from build123d import *

# Parameters (mm, degrees)
SKETCH1_W               = 44.45
SKETCH1_H               = 63.5
BOSS_EXTRUDE1_DEPTH     = 6.35
F_1_4_CLEARANCE_HOLE1_D = 6.7564
F_1_4_CLEARANCE_HOLE3_D = 6.5278


with BuildPart() as part:
    # Sketch1 → Boss-Extrude1 (new body)
    with BuildSketch(Plane(origin=(0, 0, 0), x_dir=(1, 0, 0), z_dir=(0, 1, 0))):
        Rectangle(SKETCH1_W, SKETCH1_H)
    extrude(amount=BOSS_EXTRUDE1_DEPTH)

    # 1/4 Clearance Hole1 (through all)
    with Locations(Plane(origin=(0, 6.35, 0), x_dir=(1, 0, 0), z_dir=(0, 1, 0))):
        with Locations((0, 25.4), (0, 0)):
            Hole(F_1_4_CLEARANCE_HOLE1_D / 2)

    # 1/4 Clearance Hole3 (through all)
    with Locations(Plane(origin=(0, 6.35, 0), x_dir=(1, 0, 0), z_dir=(0, 1, 0))):
        with Locations((-12.7, -22.86), (12.7, -22.86)):
            Hole(F_1_4_CLEARANCE_HOLE3_D / 2)


solid = part.part
Model file for the job. Use its own axes, mm. Give positions to 0.01 mm unless a question says otherwise; leave off trailing zeros. Write each loop counter-clockwise with the first axis right and the second up, starting at its lowest first coordinate (ties: lowest second). Pieces come first, ordered by that corner, then holes. Notation, with made-up numbers: M -11.5,70.25 L 23.5,70.25 A23 ccw 23.5,86.25 Z; hole C 53.25,4.5 d1. An arc over 180 degrees is marked long. One line per item, written item: value. Start each with the question number.
Q1. Saw through at D-D, the plane x = 0. Write the cut outline in (y, z).
Q2. Saw through at C-C, the plane y = 1.25. Write the cut outline in (x, z) (3 decimals), plus the area to 3 significant figures.
Q3. Drop a flat-ended pin along its axis: pin 1 Ø7.5 at (x, z) = (12.7, 22.86) entering from -Y. Give the stop position or say it passes through.
Q4. Two-plate mould, pull along Z, no slides. Class faces 1 (the cylindrical face through (2.681, 3.131, 2.056)), 2 (the flat face through (-5, 6.35, 0)), 3 (the flat face through (0, 3, -31.75)): +Z half, -Z half, draft (parallel to the pull), parting line (faces both ways), or undercut.
Q5. Saw through at B-B, the plane x = -12.7. Write the cut outline in (y, z).
Q6. Saw through at A-A, the plane z = -25.4. Write the cut outline in (x, y) (3 decimals), plus the area to 3 significant figures.
Q7. Probe probe 1 along X at (y, z) = (1.75, 22.86) (3 decimals); probe 2 along Z at (x, y) = (0, 3.5); probe 3 along X at (y, z) = (3, -25.4) (3 decimals). List the from-to ranges inside material, lowest first. Write a range as [from, to].
Output values:
1. outline: M 0,-31.75 L 6.35,-31.75 L 6.35,-28.78 L 0,-28.78 Z; M 0,-22.02 L 6.35,-22.02 L 6.35,-3.38 L 0,-3.38 Z; M 0,3.38 L 6.35,3.38 L 6.35,31.75 L 0,31.75 Z
2. outline: M -22.225,-31.75 L 22.225,-31.75 L 22.225,31.75 L -22.225,31.75 Z; hole C -12.7,22.86 d6.528; hole C 0,-25.4 d6.756; hole C 0,0 d6.756; hole C 12.7,22.86 d6.528
2. area: 2,680 mm²
3. pin 1: stops at y = 0
4. face 1: undercut
4. face 2: draft
4. face 3: -Z half
5. outline: M 0,-31.75 L 6.35,-31.75 L 6.35,19.6 L 0,19.6 Z; M 0,26.12 L 6.35,26.12 L 6.35,31.75 L 0,31.75 Z
6. outline: M -22.225,0 L -3.378,0 L -3.378,6.35 L -22.225,6.35 Z; M 3.378,0 L 22.225,0 L 22.225,6.35 L 3.378,6.35 Z
6. area: 239 mm²
7. probe 1: x = [-22.225, -15.964], [-9.436, 9.436], [15.964, 22.225]
7. probe 2: z = [-31.75, -28.78], [-22.02, -3.38], [3.38, 31.75]
7. probe 3: x = [-22.225, -3.378], [3.378, 22.225]
